Input: dimensioned drawing with shaded views. Units: mm. Origin: part minimum x, y, z. Give positions to 0.01 mm unless a question says otherwise; leave off trailing zeros. Write each loop counter-clockwise with the first axis right and the second up, starting at its lowest first coordinate (ties: lowest second). Pieces come first, ordered by that corner, then holes. Notation, with made-up numbers: (57, 7) - (87, 7) arc R29 cw to (87, 31) - close; hole circle Ø3 at (10, -29). An arc over 180 degrees is marked (long way). Answer as CSV lines item,"result".
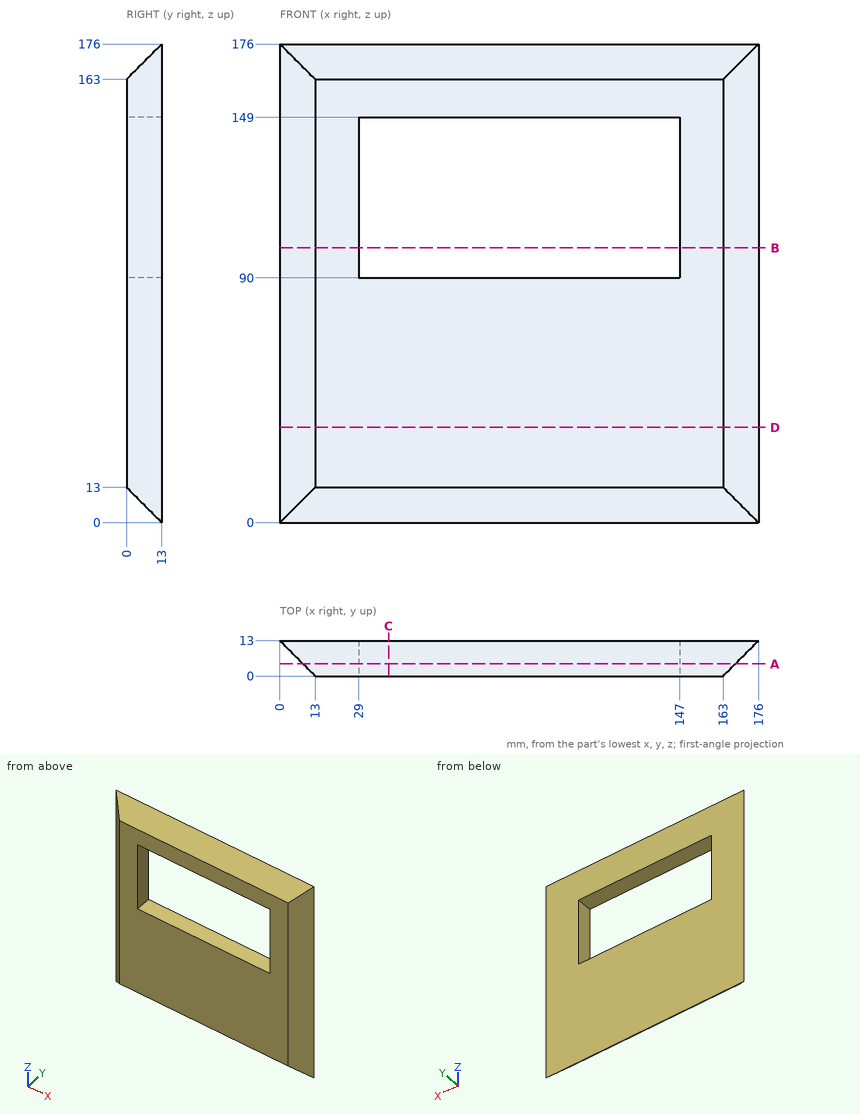
Item 1: Cut plane B-B on z = 101. Return the cut outline in (x, y).
The answers:
outline,"(0, 13) - (13, 0) - (29, 0) - (29, 13) - close; (147, 0) - (163, 0) - (176, 13) - (147, 13) - close"
Item 2: Cut plane D-D on z = 35. Return the cut outline in (x, y), plus the area to 3 significant figures.
The answers:
outline,"(0, 13) - (13, 0) - (163, 0) - (176, 13) - close"
area,"2,120 mm²"
Item 3: Cut plane C-C on x = 40. Return the cut outline in (y, z).
The answers:
outline,"(0, 13) - (13, 0) - (13, 90) - (0, 90) - close; (0, 149) - (13, 149) - (13, 176) - (0, 163) - close"
Item 4: Contact query for flat-ended pins moving along their axis: pin 1 (4 mm diameter, centred on y = 5, z = 149, fed in from +X); pin 2 (2 mm diameter, centred on x = 117.5, y = 1.5, fed in from +Z); pin 3 (3 mm diameter, centred on x = 68.5, y = 6.5, fed in from +Z). Output: stop coordinate, or through.
The answers:
pin 1,"x = 170"
pin 2,"z = 165.5"
pin 3,"z = 171"
Item 5: Cut plane A-A on y = 4.5. Return the cut outline in (x, z).
The answers:
outline,"(8.5, 8.5) - (167.5, 8.5) - (167.5, 167.5) - (8.5, 167.5) - close; hole (29, 90) - (147, 90) - (147, 149) - (29, 149) - close"
Item 6: Ray query, line 1 (Z direction, x = 74, y = 2.25); line 2 (X direction, y = 6, z = 116); line 3 (Z direction, x = 101, y = 11.5). Return the intervals inside material, ascending. Write a range as from..to.
The answers:
line 1,"10.75..90, 149..165.25"
line 2,"7..29, 147..169"
line 3,"1.5..90, 149..174.5"
